Here's how the part is built. I have some questions about the finished solid (model axes, mm). A direction names the side the tool comes from. Give positions to 0.01 mm unless a question says otherwise; leave off trailing zeros. Write each loop counter-clockwise with the first axis right and the second up, starting at its lowest first coordinate (ties: lowest second). Pieces come first, ordered by that corner, then holes. Notation, with made-up numbers: (37.5, 32.5) - (87.5, 32.5) arc R23 ccw to (87.5, 61.5) - close; hole circle Ø2 at (61, 77). An arc over 180 degrees is marked (long way). Use a Markdown table: item, result.
```python
from build123d import *

# Parameters (mm, degrees)
SIDE_DEPTH             = 2.54
COVER_DEPTH            = 44.45
FLYWHEEL_SLIT_REACH    = 107.934
MOUNT_HOLES_REACH      = 107.934
SKETCH4_R              = 3.2639
AXLE_HOLDER_HOLE_REACH = 107.934
SKETCH5_R              = 5.08


with BuildPart() as part:
    # Sketch1 → Side (new body)
    with BuildSketch(Plane.XY):
        with BuildLine():
            Line((17.780628438, -45.433815472), (42.794745364, -49.844479185))
            ThreePointArc((42.794745364, -49.844479185), (50.891612275, 42.70313309), (-41.656, 50.8))
            Line((-41.656, 50.8), (-41.656, 25.4))
            Line((-41.656, 25.4), (-39.624, 25.4))
            Line((-39.624, 25.4), (-39.624, 0))
            Line((-39.624, 0), (0, 0))
            Line((0, 0), (-6.880635392, -39.022022405))
            Line((-6.880635392, -39.022022405), (18.133481535, -43.432686118))
            Line((18.133481535, -43.432686118), (17.780628438, -45.433815472))
        make_face()
        with BuildLine():
            Line((0, 0), (-39.624, 0))
            ThreePointArc((-39.624, 0), (-30.353745014, -25.469816246), (-6.880635392, -39.022022405))
            Line((-6.880635392, -39.022022405), (0, 0))
        make_face()
    side = extrude(amount=SIDE_DEPTH)

    # Sketch2 → Cover (add)
    with BuildSketch(Plane.XY.offset(2.54)):
        with BuildLine():
            Line((-40.023319471, 48.854247114), (-41.656, 48.854247114))
            Line((-41.656, 48.854247114), (-41.656, 50.8))
            ThreePointArc((-41.656, 50.8), (50.891612275, 42.70313309), (42.794745364, -49.844479185))
            Line((42.794745364, -49.844479185), (40.878552837, -49.506602742))
            Line((40.878552837, -49.506602742), (41.162064836, -47.898726299))
            ThreePointArc((41.162064836, -47.898726299), (48.945859389, 41.070452561), (-40.023319471, 48.854247114))
        make_face()
    extrude(amount=COVER_DEPTH)

    # Mirror1: Side across plane
    add(side.mirror(Plane.XY.offset(24.765)))

    # Sketch3 → Flywheel slit (cut, up to next)
    with BuildSketch(Plane.XY.offset(49.53), mode=Mode.PRIVATE) as flywheel_slit_sk1:
        with BuildLine():
            Line((-4.081701322, 4.864382214), (-37.159500375, -22.891186772))
            Line((-37.159500375, -22.891186772), (-28.996097732, -32.6199512))
            Line((-28.996097732, -32.6199512), (4.081701322, -4.864382214))
            ThreePointArc((4.081701322, -4.864382214), (4.864382214, 4.081701322), (-4.081701322, 4.864382214))
        make_face()
    flywheel_slit_tool1 = extrude(flywheel_slit_sk1.sketch, amount=-FLYWHEEL_SLIT_REACH, mode=Mode.PRIVATE) & part.part
    add(flywheel_slit_tool1.solids().sort_by_distance((-14.612688, -12.261501, 49.53))[0], mode=Mode.SUBTRACT)

    # Sketch4 → Mount holes (cut, up to next)
    with BuildSketch(Plane(origin=(0, 0, 0), x_dir=(-1, 0, 0), z_dir=(0, 0, -1)), mode=Mode.PRIVATE) as mount_holes_sk1:
        with Locations((-2.116217682, -33.531680079)):
            Circle(SKETCH4_R)
    mount_holes_tool1 = extrude(mount_holes_sk1.sketch, amount=-MOUNT_HOLES_REACH, mode=Mode.PRIVATE) & part.part
    # Sketch4 → Mount holes (cut, up to next)
    with BuildSketch(Plane(origin=(0, 0, 0), x_dir=(-1, 0, 0), z_dir=(0, 0, -1)), mode=Mode.PRIVATE) as mount_holes_sk2:
        with Locations((33.277492898, 10.173950581)):
            Circle(SKETCH4_R)
    mount_holes_tool2 = extrude(mount_holes_sk2.sketch, amount=-MOUNT_HOLES_REACH, mode=Mode.PRIVATE) & part.part
    add(mount_holes_tool1.solids().sort_by_distance((2.116218, -33.53168, 0))[0], mode=Mode.SUBTRACT)
    add(mount_holes_tool2.solids().sort_by_distance((-33.277493, 10.173951, 0))[0], mode=Mode.SUBTRACT)

    # Sketch5 → Axle Holder Hole (cut, up to next)
    with BuildSketch(Plane(origin=(0, 0, 0), x_dir=(-1, 0, 0), z_dir=(0, 0, -1)), mode=Mode.PRIVATE) as axle_holder_hole_sk1:
        Circle(SKETCH5_R)
    axle_holder_hole_tool1 = extrude(axle_holder_hole_sk1.sketch, amount=-AXLE_HOLDER_HOLE_REACH, mode=Mode.PRIVATE) & part.part
    add(axle_holder_hole_tool1.solids().sort_by_distance((0, 0, 0))[0], mode=Mode.SUBTRACT)


solid = part.part
```
Item 1: Thinking about a two-plate mould opening in Z: for faces 5 (the flat face through (12, 9, 49.53)), 6 (the cylindrical face through (49.827, 39.997, 24.454)), 7 (the cylindrical face through (-17.124, -35.733, 48.278)), which applies, +Z half, -Z half, draft (parallel to the pull), parting line (faces both ways), or undercut?
Values:
| item | result |
|---|---|
| face 5 | +Z half |
| face 6 | undercut |
| face 7 | draft |
Item 2: If we section it at A-A, the plane y = -16: Write out the boundary of the cut face in (x, z), plus the area to 3 significant figures.
Values:
| item | result |
|---|---|
| outline | (-36.25, 0) - (64.16, 0) - (64.16, 49.53) - (-9.19, 49.53) - (-9.19, 46.99) - (61.53, 46.99) - (61.53, 2.54) - (-36.25, 2.54) - close; (-36.25, 46.99) - (-28.95, 46.99) - (-28.95, 49.53) - (-36.25, 49.53) - close |
| area | 577 mm2 |
Item 3: If we section it at B-B, the plane x = -8.5: Write out the boundary of the cut face in (y, z), plus the area to 3 significant figures.
Values:
| item | result |
|---|---|
| outline | (-38.7, 0) - (65.54, 0) - (65.54, 49.53) - (1.16, 49.53) - (1.16, 46.99) - (62.97, 46.99) - (62.97, 2.54) - (-38.7, 2.54) - close; (-38.7, 46.99) - (-15.42, 46.99) - (-15.42, 49.53) - (-38.7, 49.53) - close |
| area | 601 mm2 |
Item 4: For faces 1 (the cylindrical face through (2.541, -30.296, 1.252)), 2 (the flat face through (-39.624, 13, 1)), 3 (the flat face through (-41.656, 49.4, 24.9)), 4 (the flat face through (-18.85, -7.53, 48.28)), which set-ups out of +Z, -Z, +X, -X, +Y, -Y let a thin tool reach every point of the face, with its end or its side?
Values:
| item | result |
|---|---|
| face 1 | -Z |
| face 2 | +Z, -Z, -X, -Y |
| face 3 | +Z, -Z, -X, +Y, -Y |
| face 4 | +Z |
Item 5: If we section it at D-D, the plane x = 50: Write out the boundary of the cut face in (y, z), plus the area to 3 significant figures.
Values:
| item | result |
|---|---|
| outline | (-42.79, 0) - (43.74, 0) - (43.74, 49.53) - (-42.79, 49.53) - close; hole (-38.82, 2.54) - (39.78, 2.54) - (39.78, 46.99) - (-38.82, 46.99) - close |
| area | 792 mm2 |
Item 6: I need wall thicknesses on line 1 along Z through (x, y) = (-24, 16); line 2 along X through (y, z) = (55, 8.5); line 3 along Y through (x, z) = (0, 0.8). Which ranges of each line are inside material? Lowest first, please. Write a range as [from, to].
Values:
| item | result |
|---|---|
| line 1 | z = [0, 2.54], [46.99, 49.53] |
| line 2 | x = [-36.07, -31.3], [32.43, 37.21] |
| line 3 | y = [-40.24, -36.02], [-31.05, -5.08], [5.08, 66.17] |
Item 7: Will these pins go through, and if not, where does the flat tip stop? pin 1 Ø8 at (x, z) = (-12.5, 11.5) entering from +Y; pin 2 Ø1.5 at (y, z) = (-32.5, 22.5) entering from -X; pin 3 Ø2 at (x, z) = (30, 8) entering from -Y.
Values:
| item | result |
|---|---|
| pin 1 | stops at y = 65.54 |
| pin 2 | stops at x = 53.96 |
| pin 3 | stops at y = 55.81 |
